Geometry check sheet. Reference: drawing and pictorial views, mm from the part's lowest x, y, z. Give positions to 0.01 mm unless a question says otherwise; leave off trailing zeros. Order: outer loops, then holes, each group sorted by start corner. A loop starts at its lowest first (then second) coordinate and runs counter-clockwise, first axis right, second up. Notation, with made-up numbers: (-34.75, 32) -> (24.25, 32) arc R21 cw to (24.25, 69) -> close; hole circle Ø3 at (34, -25.5). An arc over 180 degrees is marked (long way). Write each question's results on one line, items separated by ' | '. Start each with the question number.
1. Cross-section at A-A, the plane x = 60. Enter the section's corners in (y, z) (1 decimal), then the cut area to 3 significant figures.
2. Material ranges on L1, parallel to Z at x = 50.8, y = 6.25; L2, parallel to Z at x = 48, y = 7.25; L3, parallel to X at y = 6, z = 38, recorded low to high. Write a range as from..to.
3. Cross-section at B-B, the plane z = 38.5. Enter the section's corners in (x, y) (1 decimal).
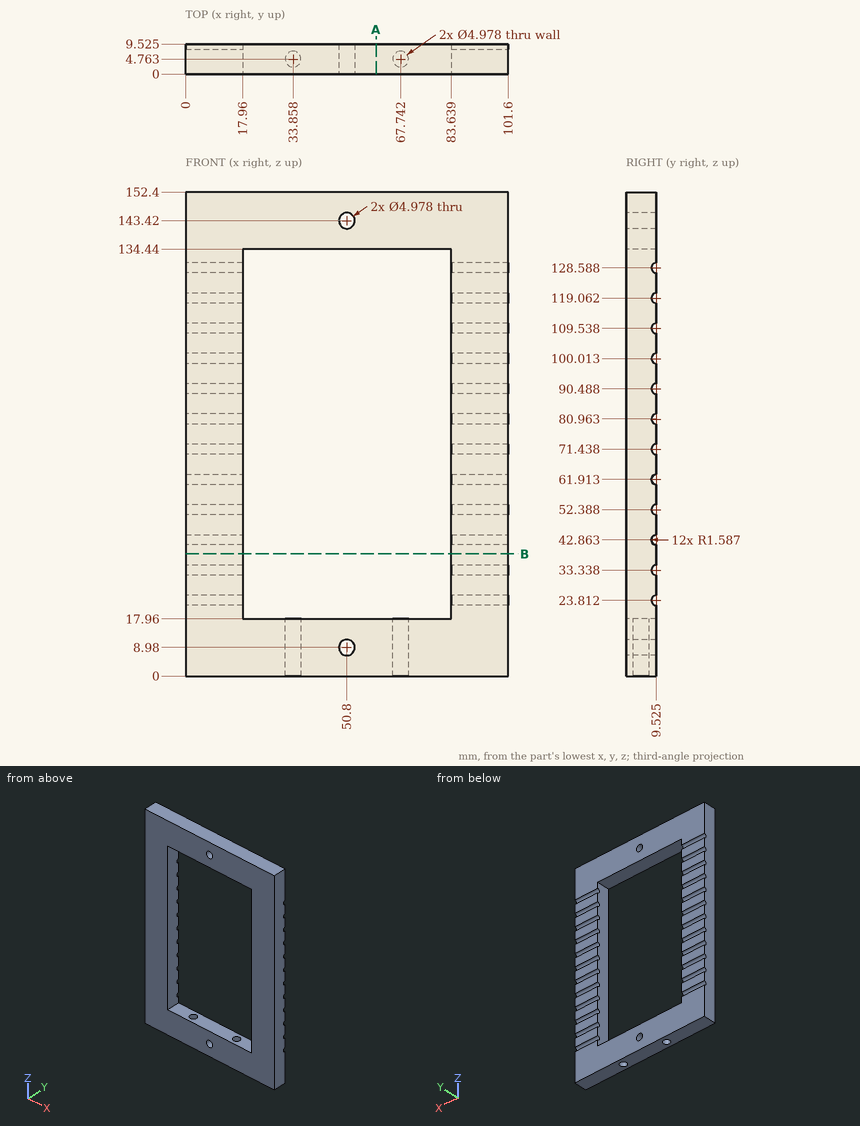
Results below:
1) outline: (0, 0) -> (9.5, 0) -> (9.5, 18) -> (0, 18) -> close; (0, 134.4) -> (9.5, 134.4) -> (9.5, 152.4) -> (0, 152.4) -> close | area: 342 mm²
2) L1: z = 0..6.49, 11.47..17.96, 134.44..140.93, 145.91..152.4 | L2: z = 0..17.96, 134.44..152.4 | L3: x = 0..17.96, 83.64..101.6
3) outline: (0, 0) -> (18, 0) -> (18, 9.5) -> (0, 9.5) -> close; (83.6, 0) -> (101.6, 0) -> (101.6, 9.5) -> (83.6, 9.5) -> close
